Geometry check sheet. Reference: the model listing, model coordinates, mm. A direction names the side the tool comes from. Coordinates: 2 decimals unless noted, no trailing zeros. Write each loop counter-clockwise with the first axis right and the second up, starting at its lowest first coordinate (ties: lowest second). Pieces come first, ordered by that corner, then holes. Notation, with made-up numbers: (87.5, 32) -> (110.5, 32) arc R18 ccw to (110.5, 47) -> close; hole circle Ø1 at (65, 54). An arc over 180 degrees is marked (long way). One line per question, with ' | ' between items.
from build123d import *

# Parameters (mm, degrees)
BOSS_EXTRUDE1_DEPTH = 7
SKETCH2_R           = 4
CUT_EXTRUDE1_DEPTH  = 4
SKETCH3_R           = 2.25
CUT_EXTRUDE2_DEPTH  = 4
SKETCH4_R           = 17
BOSS_EXTRUDE2_DEPTH = 8
SKETCH5_R           = 5
CUT_EXTRUDE3_DEPTH  = 15
FILLET3_R           = 1


with BuildPart() as part:
    # Sketch1 → Boss-Extrude1 (new body)
    with BuildSketch(Plane.XY):
        with BuildLine():
            Line((-14.849242405, -14.849242405), (-25.688984099, -4.009500711))
            ThreePointArc((-25.688984099, -4.009500711), (-26, 0), (-25.688984099, 4.009500711))
            Line((-25.688984099, 4.009500711), (-14.849242405, 14.849242405))
            Line((-14.849242405, 14.849242405), (-4.009500711, 25.688984099))
            ThreePointArc((-4.009500711, 25.688984099), (0, 26), (4.009500711, 25.688984099))
            Line((4.009500711, 25.688984099), (14.849242405, 14.849242405))
            Line((14.849242405, 14.849242405), (25.688984099, 4.009500711))
            ThreePointArc((25.688984099, 4.009500711), (26, 0), (25.688984099, -4.009500711))
            Line((25.688984099, -4.009500711), (14.849242405, -14.849242405))
            Line((14.849242405, -14.849242405), (4.009500711, -25.688984099))
            ThreePointArc((4.009500711, -25.688984099), (0, -26), (-4.009500711, -25.688984099))
            Line((-4.009500711, -25.688984099), (-14.849242405, -14.849242405))
        make_face()
    extrude(amount=BOSS_EXTRUDE1_DEPTH)

    # Sketch2 → Cut-Extrude1 (cut)
    with BuildSketch(Plane(origin=(0, 0, 0), x_dir=(-1, 0, 0), z_dir=(0, 0, -1))):
        with Locations((0, 21)):
            Circle(SKETCH2_R)
        with Locations((-21, 0)):
            Circle(SKETCH2_R)
        with Locations((0, -21)):
            Circle(SKETCH2_R)
        with Locations((21, 0)):
            Circle(SKETCH2_R)
    extrude(amount=-CUT_EXTRUDE1_DEPTH, mode=Mode.SUBTRACT)

    # Sketch3 → Cut-Extrude2 (cut)
    with BuildSketch(Plane(origin=(0, 0, 4), x_dir=(-1, 0, 0), z_dir=(0, 0, -1))):
        with Locations((0, 21)):
            Circle(SKETCH3_R)
        with Locations((-21, 0)):
            Circle(SKETCH3_R)
        with Locations((21, 0)):
            Circle(SKETCH3_R)
        with Locations((0, -21)):
            Circle(SKETCH3_R)
    extrude(amount=-CUT_EXTRUDE2_DEPTH, mode=Mode.SUBTRACT)

    # Sketch4 → Boss-Extrude2 (add)
    with BuildSketch(Plane.XY.offset(7)):
        Circle(SKETCH4_R)
    extrude(amount=BOSS_EXTRUDE2_DEPTH)

    # Sketch5 → Cut-Extrude3 (cut)
    with BuildSketch(Plane.XY.offset(15)):
        Circle(SKETCH5_R)
    extrude(amount=-CUT_EXTRUDE3_DEPTH, mode=Mode.SUBTRACT)

    # Fillet3
    fillet3_edges = [part.edges().sort_by_distance(p)[0] for p in [
        (-17, 0, 7),
        (-17, 0, 15),
        (-5, 0, 15),
    ]]
    fillet(fillet3_edges, radius=FILLET3_R)


solid = part.part
1. Cross-section at B-B on x = 21. Record the boundary of the cut face in (y, z), and give its area (3 significant figures).
Worked answers:
outline: (-8.7, 0) -> (-4, 0) -> (-4, 4) -> (-2.25, 4) -> (-2.25, 7) -> (-8.7, 7) -> close; (2.25, 4) -> (4, 4) -> (4, 0) -> (8.7, 0) -> (8.7, 7) -> (2.25, 7) -> close | area: 76.3 mm²
2. Mould release check, pull along Y, two halves, no side actions. Record for faces 3 (the face through (-14.7, -15, 3.5)), 4 (the face through (0.521, -17.034, 1.972)), 5 (the face through (5.9, 17.5, 7)): released by +Y, released by -Y, zero draft, split by the parting line, or undercut.
Worked answers:
face 3: released by -Y | face 4: undercut | face 5: zero draft
3. Tool access check on faces 1 (the face through (0.488, 18.804, 5.479)), 2 (the face through (-17.8, -2.4, 2)). Record the directions out of +Z, -Z, +X, -X, +Y, -Y that give a thin tool (end or side, any length) a straight path to the whole face; none if there is none.
Worked answers:
face 1: +Z, -Z | face 2: -Z
4. Cross-section at D-D on z = 10. Record the boundary of the cut face in (x, y).
Worked answers:
outline: circle Ø34 at (0, 0); hole circle Ø10 at (0, 0)
5. Material ranges on line 1 (Y direction, x = 0, z = 2.25); line 2 (Y direction, x = 21, z = 2.25); line 3 (X direction, y = -23, z = 2), recorded low to high. Write a range as from..to.
Worked answers:
line 1: -26..-25, -17..-5, 5..17, 25..26 | line 2: -8.7..-4, 4..8.7 | line 3: -6.7..-3.46, 3.46..6.7
6. Go/stop test with flat-tipped pins: P1, Ø5, axis at x = -21, y = 0, coming from the +Z side; P2, Ø3, axis at y = 4.5, z = 13.5, coming from the -X side; P3, Ø2.5, axis at x = 21, y = 0, coming from the -Z side; P4, Ø4, axis at y = -6.5, z = 7, coming from the +X side. Record where each tip stops, or that it passes through.
Worked answers:
P1: z = 7 | P2: x = -16.73 | P3: through | P4: x = 25.2
7. Cross-section at A-A on z = 3. Record the boundary of the cut face in (x, y), and give its area (3 significant figures).
Worked answers:
outline: (-25.69, -4.01) -> (-4.01, -25.69) arc R26 ccw to (4.01, -25.69) -> (25.69, -4.01) arc R26 ccw to (25.69, 4.01) -> (4.01, 25.69) arc R26 ccw to (-4.01, 25.69) -> (-25.69, 4.01) arc R26 ccw to start; hole circle Ø8 at (-21, 0); hole circle Ø10 at (0, 0); hole circle Ø8 at (0, -21); hole circle Ø8 at (0, 21); hole circle Ø8 at (21, 0) | area: 1,430 mm²
